Could you check a few things on this model? Use its own coordinates, in mm. Give positions to 0.01 mm unless a question says otherwise; leave off trailing zeros. Loops run counter-clockwise (first coordinate to the right, second up) from the corner with the lowest first, then second, coordinate; pieces in that order, holes last. Notation, with made-up numbers: M 31.25,-20 L 55.25,-20 A21 cw 55.25,16 Z; hole C 37,1 d6. An arc over 180 degrees is marked long. Use CSV: the item, a comma, the result in double quotes.
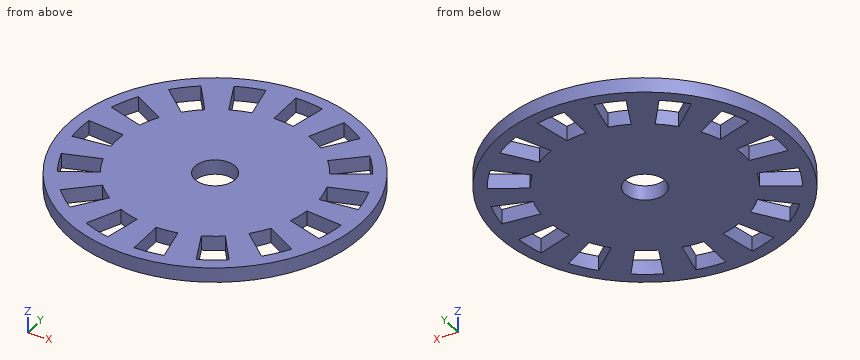
```python
from build123d import *

# Parameters (mm, degrees)
F0_R     = 30
F0_R_2   = 4.1
F1_DEPTH = 3


with BuildPart() as f1:
    # F0 (on Top) → F1 (new body)
    with BuildSketch(Plane.XY):
        Circle(F0_R)
        with BuildLine():
            ThreePointArc((-16.164094, -22.247967), (-18.401092, -20.436483), (-20.436483, -18.401092))
            Line((-20.436483, -18.401092), (-14.862897, -13.382612))
            ThreePointArc((-14.862897, -13.382612), (-13.382612, -14.862897), (-11.755705, -16.18034))
            Line((-11.755705, -16.18034), (-16.164094, -22.247967))
        make_face(mode=Mode.SUBTRACT)
        with BuildLine():
            ThreePointArc((-5.717571, -26.899059), (-8.497967, -26.154054), (-11.185258, -25.1225))
            Line((-11.185258, -25.1225), (-8.134733, -18.270909))
            ThreePointArc((-8.134733, -18.270909), (-6.18034, -19.02113), (-4.158234, -19.562952))
            Line((-4.158234, -19.562952), (-5.717571, -26.899059))
        make_face(mode=Mode.SUBTRACT)
        with BuildLine():
            ThreePointArc((-23.815699, -13.75), (-25.1225, -11.185258), (-26.154054, -8.497967))
            Line((-26.154054, -8.497967), (-19.02113, -6.18034))
            ThreePointArc((-19.02113, -6.18034), (-18.270909, -8.134733), (-17.320508, -10))
            Line((-17.320508, -10), (-23.815699, -13.75))
        make_face(mode=Mode.SUBTRACT)
        with BuildLine():
            ThreePointArc((5.717571, -26.899059), (2.874533, -27.349352), (0, -27.5))
            Line((0, -27.5), (0, -20))
            ThreePointArc((0, -20), (2.090569, -19.890438), (4.158234, -19.562952))
            Line((4.158234, -19.562952), (5.717571, -26.899059))
        make_face(mode=Mode.SUBTRACT)
        with BuildLine():
            ThreePointArc((16.164094, -22.247967), (13.75, -23.815699), (11.185258, -25.1225))
            Line((11.185258, -25.1225), (8.134733, -18.270909))
            ThreePointArc((8.134733, -18.270909), (10, -17.320508), (11.755705, -16.18034))
            Line((11.755705, -16.18034), (16.164094, -22.247967))
        make_face(mode=Mode.SUBTRACT)
        with BuildLine():
            ThreePointArc((23.815699, -13.75), (22.247967, -16.164094), (20.436483, -18.401092))
            Line((20.436483, -18.401092), (14.862897, -13.382612))
            ThreePointArc((14.862897, -13.382612), (16.18034, -11.755705), (17.320508, -10))
            Line((17.320508, -10), (23.815699, -13.75))
        make_face(mode=Mode.SUBTRACT)
        with BuildLine():
            ThreePointArc((27.349352, -2.874533), (26.899059, -5.717571), (26.154054, -8.497967))
            Line((26.154054, -8.497967), (19.02113, -6.18034))
            ThreePointArc((19.02113, -6.18034), (19.562952, -4.158234), (19.890438, -2.090569))
            Line((19.890438, -2.090569), (27.349352, -2.874533))
        make_face(mode=Mode.SUBTRACT)
        with BuildLine():
            ThreePointArc((-27.349352, -2.874533), (-27.5, 0), (-27.349352, 2.874533))
            Line((-27.349352, 2.874533), (-19.890438, 2.090569))
            ThreePointArc((-19.890438, 2.090569), (-20, 0), (-19.890438, -2.090569))
            Line((-19.890438, -2.090569), (-27.349352, -2.874533))
        make_face(mode=Mode.SUBTRACT)
        with BuildLine():
            ThreePointArc((-26.154054, 8.497967), (-25.1225, 11.185258), (-23.815699, 13.75))
            Line((-23.815699, 13.75), (-17.320508, 10))
            ThreePointArc((-17.320508, 10), (-18.270909, 8.134733), (-19.02113, 6.18034))
            Line((-19.02113, 6.18034), (-26.154054, 8.497967))
        make_face(mode=Mode.SUBTRACT)
        with BuildLine():
            ThreePointArc((-20.436483, 18.401092), (-18.401092, 20.436483), (-16.164094, 22.247967))
            Line((-16.164094, 22.247967), (-11.755705, 16.18034))
            ThreePointArc((-11.755705, 16.18034), (-13.382612, 14.862897), (-14.862897, 13.382612))
            Line((-14.862897, 13.382612), (-20.436483, 18.401092))
        make_face(mode=Mode.SUBTRACT)
        with BuildLine():
            ThreePointArc((-11.185258, 25.1225), (-8.497967, 26.154054), (-5.717571, 26.899059))
            Line((-5.717571, 26.899059), (-4.158234, 19.562952))
            ThreePointArc((-4.158234, 19.562952), (-6.18034, 19.02113), (-8.134733, 18.270909))
            Line((-8.134733, 18.270909), (-11.185258, 25.1225))
        make_face(mode=Mode.SUBTRACT)
        Circle(F0_R_2, mode=Mode.SUBTRACT)
        with BuildLine():
            ThreePointArc((26.154054, 8.497967), (26.899059, 5.717571), (27.349352, 2.874533))
            Line((27.349352, 2.874533), (19.890438, 2.090569))
            ThreePointArc((19.890438, 2.090569), (19.562952, 4.158234), (19.02113, 6.18034))
            Line((19.02113, 6.18034), (26.154054, 8.497967))
        make_face(mode=Mode.SUBTRACT)
        with BuildLine():
            ThreePointArc((20.436483, 18.401092), (22.247967, 16.164094), (23.815699, 13.75))
            Line((23.815699, 13.75), (17.320508, 10))
            ThreePointArc((17.320508, 10), (16.18034, 11.755705), (14.862897, 13.382612))
            Line((14.862897, 13.382612), (20.436483, 18.401092))
        make_face(mode=Mode.SUBTRACT)
        with BuildLine():
            ThreePointArc((11.185258, 25.1225), (13.75, 23.815699), (16.164094, 22.247967))
            Line((16.164094, 22.247967), (11.755705, 16.18034))
            ThreePointArc((11.755705, 16.18034), (10, 17.320508), (8.134733, 18.270909))
            Line((8.134733, 18.270909), (11.185258, 25.1225))
        make_face(mode=Mode.SUBTRACT)
        with BuildLine():
            Line((0, 20), (0, 27.5))
            ThreePointArc((0, 27.5), (2.874533, 27.349352), (5.717571, 26.899059))
            Line((5.717571, 26.899059), (4.158234, 19.562952))
            ThreePointArc((4.158234, 19.562952), (2.090569, 19.890438), (0, 20))
        make_face(mode=Mode.SUBTRACT)
    extrude(amount=F1_DEPTH)


solid = f1.part
```
1. I want a section at C-C, the plane z = 1.6. Give the number of separate pieces and of enclosed holes in the cut face, then the cut area to 3 significant figures.
Outcome:
separate pieces,"1"
enclosed holes,"16"
area,"2,220 mm2"
2. I'm going to push flat-ended pins straight in: pin 1 Ø0.9 at (y, z) = (22, 2) entering from +X; pin 2 Ø0.9 at (y, z) = (-23.5, 1) entering from +X. Where does each tip first touch, or does it pass through?
Outcome:
pin 1,"x = 20.87"
pin 2,"x = 19.2"
3. Please list where these lines run through material, in increasing order: line 1 (X direction, y = 14, z = 1.35); line 2 (X direction, y = -3.5, z = 1.15); line 3 (Y direction, x = 9, z = 2.95).
Outcome:
line 1,"-26.53 to -15.55, -14.28 to 15.55, 23.67 to 26.53"
line 2,"-29.8 to -2.14, 2.14 to 19.69, 27.28 to 29.8"
line 3,"-28.62 to -20.21, -17.86 to 17.86, 20.21 to 28.62"
4. I want a section at A-A, the plane y = 0. List the corners of the cut face in (x, z) for me.
Outcome:
outline,"M -30,0 L -27.5,0 L -27.5,3 L -30,3 Z; M -20,0 L -4.1,0 L -4.1,3 L -20,3 Z; M 4.1,0 L 30,0 L 30,3 L 4.1,3 Z"
5. I want a section at B-B, the plane y = 21.5. List the corners of the cut face in (x, z) for me, then the cut area to 3 significant figures.
Outcome:
outline,"M -20.92,0 L -17.15,0 L -17.15,3 L -20.92,3 Z; M -15.62,0 L -9.57,0 L -9.57,3 L -15.62,3 Z; M -4.57,0 L 0,0 L 0,3 L -4.57,3 Z; M 4.57,0 L 9.57,0 L 9.57,3 L 4.57,3 Z; M 15.62,0 L 20.92,0 L 20.92,3 L 15.62,3 Z"
area,"74.1 mm2"
6. I want a section at D-D, the plane y = 12. List the corners of the cut face in (x, z) for me.
Outcome:
outline,"M -27.5,0 L -24.74,0 L -24.74,3 L -27.5,3 Z; M -20.78,0 L 16,0 L 16,3 L -20.78,3 Z; M 20.78,0 L 27.5,0 L 27.5,3 L 20.78,3 Z"
